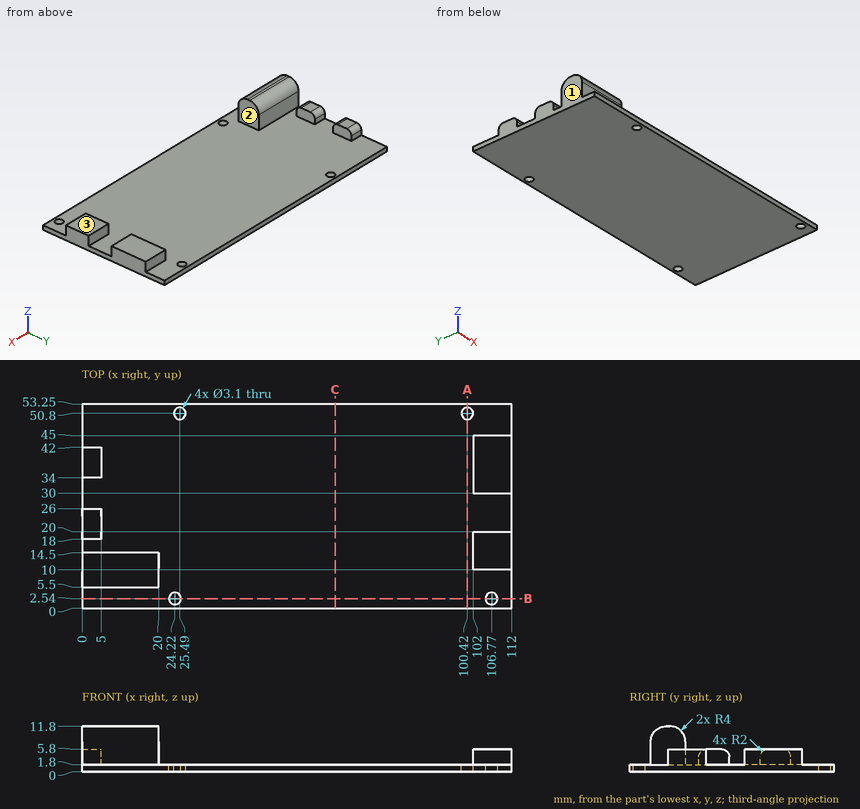
Could you check a few things on this drawing? It's one solid part, dimensions in mm from its lowest x, y, z. Coordinates: 2 decimals unless noted, no trailing zeros. Write each loop counter-clockwise with the first axis right and the second up, starting at its lowest first coordinate (ties: lowest second). Pieces come first, ordered by that corner, then holes.
1) If we section it at B-B (y = 2.54): List the corners of the cut face in (x, z) for me.
Filled in:
outline: (0, 0) - (22.67, 0) - (22.67, 1.8) - (0, 1.8) - close; (25.77, 0) - (105.22, 0) - (105.22, 1.8) - (25.77, 1.8) - close; (108.32, 0) - (112, 0) - (112, 1.8) - (108.32, 1.8) - close
2) I'm going to push flat-ended pins straight in: pin 1 (2 mm diameter, centred on x = 2, y = 21, fed in from +Z); pin 2 (4.5 mm diameter, centred on y = 8, z = 8, fed in from +X); pin 3 (1.2 mm diameter, centred on x = 105.5, z = 4, fed in from -Y); pin 4 (1 mm diameter, centred on y = 15, z = 10.5, fed in from -X). Where does each tip first touch, or does it pass through?
Filled in:
pin 1: stops at z = 5.8
pin 2: stops at x = 20
pin 3: stops at y = 10
pin 4: passes through
3) If I drill on line 1 (X direction, y = 2.54, z = 1.1); line 2 (Y direction, x = 100.42, z = 0.6); line 3 (Z direction, x = 19, y = 43), over which ranges is the centre line in solid material (lowest first)?
Filled in:
line 1: x = 0 to 22.67, 25.77 to 105.22, 108.32 to 112
line 2: y = 0 to 49.25, 52.35 to 53.25
line 3: z = 0 to 1.8
4) If we section it at A-A (x = 100.42): List the corners of the cut face in (y, z) for me, plus the area to 3 significant figures.
Filled in:
outline: (0, 0) - (49.25, 0) - (49.25, 1.8) - (0, 1.8) - close; (52.35, 0) - (53.25, 0) - (53.25, 1.8) - (52.35, 1.8) - close
area: 90.3 mm2
5) Thinking about a two-plate mould opening in X: for the marked faces 1, 2 and 3, which applies, +X half, -X half, draft (parallel to the pull), parting line (faces both ways), or undercut?
Filled in:
face 1: -X half
face 2: undercut
face 3: draft
6) If we section it at C-C (x = 66): List the corners of the cut face in (y, z) for me.
Filled in:
outline: (0, 0) - (53.25, 0) - (53.25, 1.8) - (0, 1.8) - close
